Geometry check sheet. Reference: the model listing, model coordinates, mm. Face numbers are marked on the shaded views. A direction names the side the tool comes from. Round coordinates to 2 decimals unless told otherwise and drop trailing zeros. Order: outer loops, then holes, each group sorted by start corner. A loop starts at its lowest first (then second) coordinate and runs counter-clockwise, first axis right, second up.
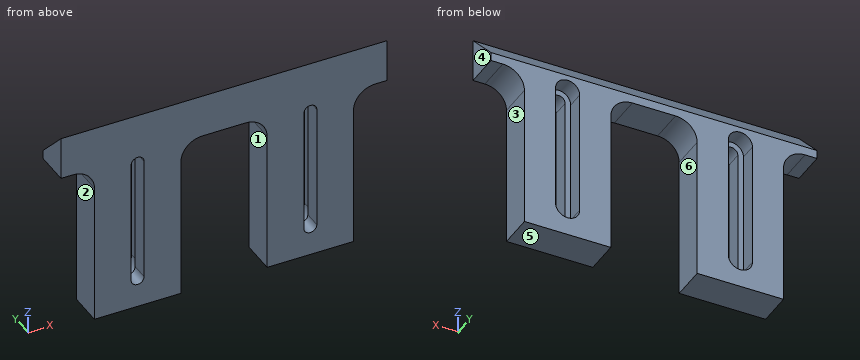
```python
from build123d import *

# Parameters (mm, degrees)
BOSS_EXTRUDE1_DEPTH = 8
CUT_EXTRUDE2_REACH  = 92.908
SKETCH5_W           = 20
SKETCH5_H           = 38
SKETCH5_W_2         = 7.75
CUT_EXTRUDE3_DEPTH  = 10
FILLET1_R           = 5
CHAMFER1_SIZE       = 10
CUT_EXTRUDE4_DEPTH  = 4


with BuildPart() as part:
    # Sketch1 → Boss-Extrude1 (new body)
    with BuildSketch(Plane(origin=(0, 0, 0), x_dir=(1, 0, 0), z_dir=(0, 1, 0))):
        Polygon((0, 0), (0, 50), (75.5, 50), (75.5, 0), (37.75, 0), align=None)
    extrude(amount=BOSS_EXTRUDE1_DEPTH)

    # Sketch4 → Cut-Extrude2 (cut, up to next)
    with BuildSketch(Plane(origin=(0, 8, 0), x_dir=(1, 0, 0), z_dir=(0, 1, 0)), mode=Mode.PRIVATE) as cut_extrude2_sk1:
        with BuildLine():
            Line((19.25, 43), (19.25, 14))
            ThreePointArc((19.25, 14), (17.75, 12.5), (16.25, 14))
            Line((16.25, 14), (16.25, 43))
            ThreePointArc((16.25, 43), (17.75, 44.5), (19.25, 43))
        make_face()
    cut_extrude2_tool1 = extrude(cut_extrude2_sk1.sketch, amount=-CUT_EXTRUDE2_REACH, mode=Mode.PRIVATE) & part.part
    # Sketch4 → Cut-Extrude2 (cut, up to next)
    with BuildSketch(Plane(origin=(0, 8, 0), x_dir=(1, 0, 0), z_dir=(0, 1, 0)), mode=Mode.PRIVATE) as cut_extrude2_sk2:
        with BuildLine():
            Line((59.25, 43), (59.25, 14))
            ThreePointArc((59.25, 14), (57.75, 12.5), (56.25, 14))
            Line((56.25, 14), (56.25, 43))
            ThreePointArc((56.25, 43), (57.75, 44.5), (59.25, 43))
        make_face()
    cut_extrude2_tool2 = extrude(cut_extrude2_sk2.sketch, amount=-CUT_EXTRUDE2_REACH, mode=Mode.PRIVATE) & part.part
    add(cut_extrude2_tool1.solids().sort_by_distance((17.75, 8, -28.5))[0], mode=Mode.SUBTRACT)
    add(cut_extrude2_tool2.solids().sort_by_distance((57.75, 8, -28.5))[0], mode=Mode.SUBTRACT)

    # Sketch5 → Cut-Extrude3 (cut)
    with BuildSketch(Plane(origin=(0, 8, 0), x_dir=(1, 0, 0), z_dir=(0, 1, 0))):
        with Locations((37.75, 31)):
            Rectangle(SKETCH5_W, SKETCH5_H)
        with Locations((71.625, 31)):
            Rectangle(SKETCH5_W_2, SKETCH5_H)
        with Locations((3.875, 31)):
            Rectangle(SKETCH5_W_2, SKETCH5_H)
    extrude(amount=-CUT_EXTRUDE3_DEPTH, mode=Mode.SUBTRACT)

    # Fillet1
    fillet1_edges = [part.edges().sort_by_distance(p)[0] for p in [
        (27.75, 4, -12),
        (47.75, 4, -12),
        (7.75, 4, -12),
        (67.75, 4, -12),
    ]]
    fillet(fillet1_edges, radius=FILLET1_R)

    # Chamfer1
    # the kernel refuses this chamfer: 10 mm, written as the material it takes off along each edge
    with BuildSketch(Plane(origin=(101.21682988, 8, 0), x_dir=(0, -0.9996219169112968, 0.027495876610586372), z_dir=(-1, 0, 0))) as chamfer1_piece_1:
        Polygon((CHAMFER1_SIZE * 0.999621916911, -CHAMFER1_SIZE * 0.0274958766106), (-CHAMFER1_SIZE * 0.0274958766106, -CHAMFER1_SIZE * 0.999621916911), (0, 0), align=None)
    extrude(amount=126.933659759, mode=Mode.SUBTRACT)

    # Sketch7 → Cut-Extrude4 (cut)
    with BuildSketch(Plane(origin=(0, 8, 0), x_dir=(1, 0, 0), z_dir=(0, 1, 0))):
        with BuildLine():
            Line((20.55, 43), (20.55, 14))
            ThreePointArc((20.55, 14), (17.75, 11.2), (14.95, 14))
            Line((14.95, 14), (14.95, 43))
            ThreePointArc((14.95, 43), (17.75, 45.8), (20.55, 43))
        make_face()
        with BuildLine():
            Line((60.55, 43), (60.55, 14))
            ThreePointArc((60.55, 14), (57.75, 11.2), (54.95, 14))
            Line((54.95, 14), (54.95, 43))
            ThreePointArc((54.95, 43), (57.75, 45.8), (60.55, 43))
        make_face()
    extrude(amount=-CUT_EXTRUDE4_DEPTH, mode=Mode.SUBTRACT)


solid = part.part
```
(1) Sectioned sample at D-D, the plane x = 69. Record the cut outline in (y, z), and give its area (3 significant figures).
Returned:
outline: (0, -13.69) - (8, -13.69) - (8, -10) - (0, -2) - close
area: 61.5 mm2
(2) Material ranges on line 1 (X direction, y = 1.75, z = -34.5); line 2 (X direction, y = 6.5, z = -42); line 3 (Z direction, x = 27.5, y = 5.25), recorded low to high.
Returned:
line 1: x = 7.75 to 16.25, 19.25 to 27.75, 47.75 to 56.25, 59.25 to 67.75
line 2: x = 7.75 to 14.95, 20.55 to 27.75, 47.75 to 54.95, 60.55 to 67.75
line 3: z = -50 to -7.25
(3) Depth check by flat-ended pin: P1, Ø2.5, axis at y = 3, z = -27.5, coming from the +X side; P2, Ø4, axis at y = 3.5, z = -33.5, coming from the -X side; P3, Ø1.7, axis at x = 18, z = -21, coming from the +Y side; P4, Ø1.5, axis at y = 7, z = -11.5, coming from the -X side. Enter the tip coordinate at first touch or a pass-through.
Returned:
P1: stops at x = 67.75
P2: stops at x = 7.75
P3: passes through
P4: stops at x = 0
(4) Draft check along X on the marked faces 4, 5 and 6. Enter one of: released by +X, released by -X, zero draft, split by the parting line, or undercut.
Returned:
face 4: released by +X
face 5: zero draft
face 6: undercut
(5) Sectioned sample at A-A, the plane z = -22. Record the cut outline in (x, y), and give its area (3 significant figures).
Returned:
outline: (7.75, 0) - (16.25, 0) - (16.25, 4) - (14.95, 4) - (14.95, 8) - (7.75, 8) - close; (19.25, 0) - (27.75, 0) - (27.75, 8) - (20.55, 8) - (20.55, 4) - (19.25, 4) - close; (47.75, 0) - (56.25, 0) - (56.25, 4) - (54.95, 4) - (54.95, 8) - (47.75, 8) - close; (59.25, 0) - (67.75, 0) - (67.75, 8) - (60.55, 8) - (60.55, 4) - (59.25, 4) - close
area: 251 mm2
(6) Set-up check for the marked faces 1, 2 and 3: record each of +Z, -Z, +X, -X, +Y, -Y from which the full face is reachable in a straight line by a thin tool's end or side.
Returned:
face 1: -Z, +Y, -Y
face 2: -Z, -X, +Y, -Y
face 3: -Z, +X, +Y, -Y
(7) Sectioned sample at B-B, the plane x = 57.75. Record the cut outline in (y, z).
Returned:
outline: (0, -50) - (8, -50) - (8, -45.8) - (4, -45.8) - (4, -44.5) - (0, -44.5) - close; (0, -12.5) - (4, -12.5) - (4, -11.2) - (8, -11.2) - (8, -10) - (0, -2) - close
(8) Sectioned sample at C-C, the plane y = 2.75. Record the cut outline in (x, z), and give its area (3 significant figures).
Returned:
outline: (0, -12) - (2.75, -12) arc R5 cw to (7.75, -17) - (7.75, -50) - (27.75, -50) - (27.75, -17) arc R5 cw to (32.75, -12) - (42.75, -12) arc R5 cw to (47.75, -17) - (47.75, -50) - (67.75, -50) - (67.75, -17) arc R5 cw to (72.75, -12) - (75.5, -12) - (75.5, -4.75) - (0, -4.75) - close; hole (16.25, -43) arc R1.5 ccw to (19.25, -43) - (19.25, -14) arc R1.5 ccw to (16.25, -14) - close; hole (56.25, -43) arc R1.5 ccw to (59.25, -43) - (59.25, -14) arc R1.5 ccw to (56.25, -14) - close
area: 1,900 mm2
